```python
from build123d import *

# Parameters (mm, degrees)
BOSS_EXTRUDE1_DEPTH   = 1.5748
SKETCH10_W            = 66.47
SKETCH10_H            = 4.17478322
BOSS_EXTRUDE3_DEPTH   = 1.575
SKETCH11_W            = 66.47
SKETCH11_H            = 0.5
CUT_EXTRUDE2_DEPTH    = 140.38485176
M2_CLEARANCE_HOLE1_D  = 2.2
F_2_0MM_DOWEL_HOLE1_D = 2
SKETCH12_W            = 5
SKETCH12_H            = 51.15
BOSS_EXTRUDE4_DEPTH   = 1.575


with BuildPart() as part:
    # BPR2 PCB Outline → Boss-Extrude1 (new body)
    with BuildSketch(Plane.XY):
        with BuildLine():
            Line((56.570984325, 67.317563979), (121.040984325, 67.317563979))
            ThreePointArc((121.040984325, 67.317563979), (121.748091106, 67.02467076), (122.040984325, 66.317563979))
            Line((122.040984325, 66.317563979), (122.040984325, 7.817563979))
            ThreePointArc((122.040984325, 7.817563979), (121.748091106, 7.110457198), (121.040984325, 6.817563979))
            Line((121.040984325, 6.817563979), (103.596984325, 6.817563979))
            Line((103.596984325, 6.817563979), (83.596984325, 6.817563979))
            Line((83.596984325, 6.817563979), (55.570984325, 6.817563979))
            Line((55.570984325, 6.817563979), (55.570984325, 66.317563979))
            ThreePointArc((55.570984325, 66.317563979), (55.863877543, 67.02467076), (56.570984325, 67.317563979))
        make_face()
    extrude(amount=-BOSS_EXTRUDE1_DEPTH)

    # Sketch10 → Boss-Extrude3 (add)
    with BuildSketch(Plane.XY):
        with Locations((88.805984325, 8.904955589)):
            Rectangle(SKETCH10_W, SKETCH10_H)
    extrude(amount=-BOSS_EXTRUDE3_DEPTH)

    # Sketch11 → Cut-Extrude2 (cut, through all)
    with BuildSketch(Plane.XY):
        with Locations((88.805984325, 7.067563979)):
            Rectangle(SKETCH11_W, SKETCH11_H)
    extrude(amount=-CUT_EXTRUDE2_DEPTH, mode=Mode.SUBTRACT)

    # M2 Clearance Hole1 (through all)
    with Locations(Plane(origin=(39.260906477, 104.204612391, -6.5748), x_dir=(1, 0, 0), z_dir=(0, 0, -1))):
        with Locations((81.030077848, 88.112048412), (81.030077848, 72.537048412), (81.030077848, 64.537048412), (81.030077848, 46.962048412), (18.060077848, 46.962048412), (18.060077848, 88.112048412)):
            Hole(M2_CLEARANCE_HOLE1_D / 2)

    # Ø2.0mm Dowel Hole1 (through all)
    with Locations(Plane(origin=(39.260906477, 104.204612391, -4.6498), x_dir=(1, 0, 0), z_dir=(0, 0, -1))):
        with Locations((26.280077848, 87.962048412), (26.280077848, 43.962048412), (75.280077848, 43.962048412), (75.280077848, 87.962048412)):
            Hole(F_2_0MM_DOWEL_HOLE1_D / 2)

    # Sketch12 → Boss-Extrude4 (add, through all)
    with BuildSketch(Plane.XY):
        with Locations((53.070984325, 36.667563979)):
            Rectangle(SKETCH12_W, SKETCH12_H)
    extrude(amount=-BOSS_EXTRUDE4_DEPTH)


solid = part.part
```
Here's how the part is built. I have some questions about the finished solid (model axes, mm). A direction names the side the tool comes from. Coordinates: 2 decimals unless noted, no trailing zeros.
1) Will these pins go through, and if not, where does the flat tip stop? pin 1 (0.8 mm diameter, centred on y = 8.5, z = -1, fed in from -X); pin 2 (0.8 mm diameter, centred on x = 52.5, z = -1, fed in from +Y).
2) Which directions (+Z, -Z, +X, -X, +Y, -Y) give clear straight access to the entire face, cutting with the end or side of a thin tool? Please do faces 4 (the face through (53, 62.243, -1)), 5 (the face through (66.335, 60.851, -0.776)), 6 (the face through (55.571, 9, -1)).
3) Imagine slicing it at A-A on z = -0.35. State how many separate pieces and enclosed holes the cut face has, and give its area (3 significant figures).
4) We'd pull the mould along Z, two halves only. Please class faces 1 (the face through (86, 38, 0)), 2 (the face through (89, 40, -1.575)), 3 (the face through (121.39, 16.04, -0.78)): +Z half, -Z half, draft (parallel to the pull), parting line (faces both ways), or undercut.
5) I need wall thicknesses on line 1 (Y direction, x = 56.5, z = -0.1); line 2 (Y direction, x = 57, z = -0.75); line 3 (X direction, y = 31.5, z = -1). Which ranges of each line are inside material? Lowest first, please.
Response values:
1. pin 1: stops at x = 55.57
1. pin 2: stops at y = 62.24
2. face 4: +Z, -Z, -X, +Y
2. face 5: +Z, -Z
2. face 6: +Z, -Z, -X, -Y
3. separate pieces: 1
3. enclosed holes: 10
3. area: 4,210 mm2
4. face 1: +Z half
4. face 2: -Z half
4. face 3: draft
5. line 1: y = 7.32 to 15.36, 16.82 to 56.51, 57.97 to 67.32
5. line 2: y = 7.32 to 15.04, 17.14 to 56.19, 58.29 to 67.32
5. line 3: x = 50.57 to 119.2, 121.38 to 122.04
